Geometry: see drawing. Coordinates: mm, zero at the bounding-box minimum. A direction names the side the tool comes from. Give positions to 0.01 mm unless a question says otherwise; leave off trailing zeros. Order: outer loops, then holes, each group sorted by start corner. A loop starts at its lowest first (then second) coordinate and runs counter-clockwise, first axis right, second up. Notation, with made-up numbers: (77, -4.5) - (124, -4.5) arc R31 ccw to (124, 22.5) - close; hole circle Ø1 at (22.5, -12.5). An arc over 180 degrees is marked (long way). One line per item, written item: value. Start each with the question number.
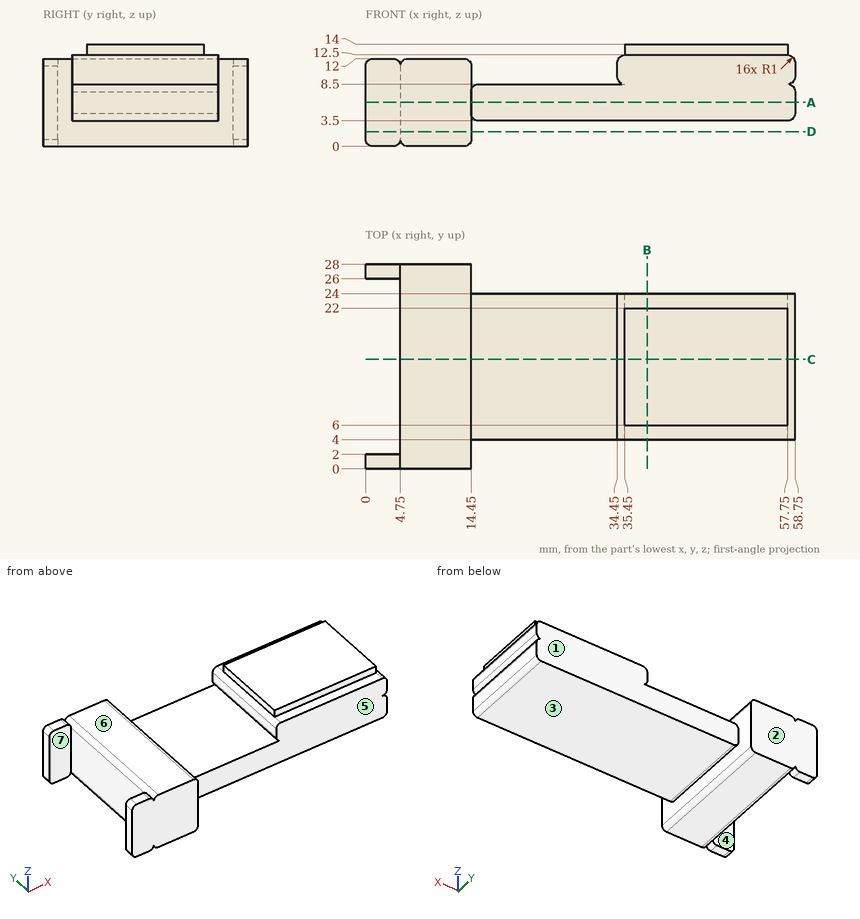
1. Contact query for flat-ended pins moving along their axis: pin 1 Ø1.6 at (x, z) = (47, 13) entering from +Y; pin 2 Ø8 at (y, z) = (9.5, 6) entering from -X; pin 3 Ø16 at (x, y) = (40.5, 19) entering from -Z. Output: stop coordinate, or through.
2. Ray query, L1, parallel to X at y = 4.5, z = 9.5; L2, parallel to X at y = 22.5, z = 6.75; L3, parallel to Y at x = 42, z = 4. Return the intervals inside material, ascending.
3. Section B-B on x = 38.5. Return the cut outline in (y, z), then the cut area to 3 significant figures.
4. Section C-C on y = 15. Return the cut outline in (x, z).
5. Section A-A on z = 6. Return the cut outline in (x, y), then the cut area to 3 significant figures.
6. Draft query along Y for the marked faces 5, 6 and 7. Return one class per face: pulls with the +Y half, pulls with the -Y half, needs draft (parallel to the pull), parting line crosses it, or undercut.
7. Set-up query: the marked faces 1, 2, 3 and 4. Return all of +Z, -Z, +X, -X, +Y, -Y with unobstructed straight access to the full face (end or side cutting, diameter ignored); none if empty.
8. Section D-D on z = 2. Return the cut outline in (x, y).
Data:
1. pin 1: stops at y = 24
1. pin 2: stops at x = 4.75
1. pin 3: stops at z = 3.5
2. L1: x = 4.75 to 14.45, 34.45 to 58.75
2. L2: x = 4.75 to 58.75
2. L3: y = 4 to 24
3. outline: (4, 3.5) - (24, 3.5) - (24, 12.5) - (22, 12.5) - (22, 14) - (6, 14) - (6, 12.5) - (4, 12.5) - close
3. area: 204 mm2
4. outline: (4.75, 1) arc R1 ccw to (5.75, 0) - (13.45, 0) arc R1 ccw to (14.45, 1) - (14.45, 4.5) arc R1 ccw to (15.45, 3.5) - (57.75, 3.5) arc R1 ccw to (58.75, 4.5) - (58.75, 7.5) arc R1 ccw to (57.75, 8.5) arc R1 ccw to (58.75, 9.5) - (58.75, 11.5) arc R1 ccw to (57.75, 12.5) - (57.75, 14) - (35.45, 14) - (35.45, 12.5) arc R1 ccw to (34.45, 11.5) - (34.45, 9.5) arc R1 ccw to (35.45, 8.5) - (15.45, 8.5) arc R1 ccw to (14.45, 7.5) - (14.45, 11) arc R1 ccw to (13.45, 12) - (5.75, 12) arc R1 ccw to (4.75, 11) - close
5. outline: (0, 0) - (14.45, 0) - (14.45, 4) - (58.75, 4) - (58.75, 24) - (14.45, 24) - (14.45, 28) - (0, 28) - (0, 26) - (4.75, 26) - (4.75, 2) - (0, 2) - close
5. area: 1,180 mm2
6. face 5: pulls with the -Y half
6. face 6: needs draft
6. face 7: undercut
7. face 1: +Z, -Z, +X, +Y
7. face 2: +Z, -Z, +X, -X, +Y
7. face 3: -Z, +X, +Y, -Y
7. face 4: +Z, -Z, -X
8. outline: (0, 0) - (14.45, 0) - (14.45, 28) - (0, 28) - (0, 26) - (4.75, 26) - (4.75, 2) - (0, 2) - close
